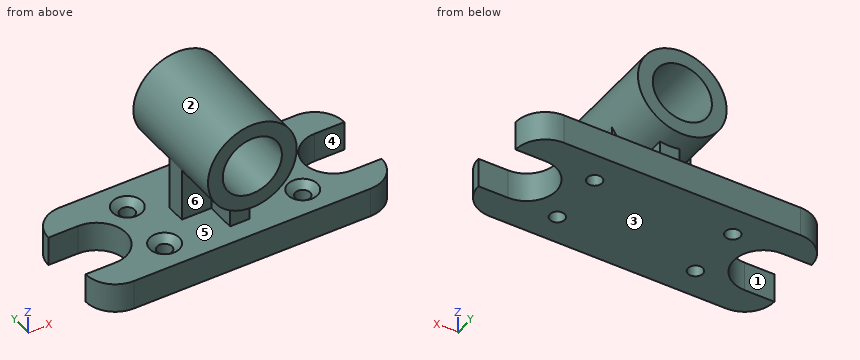
```python
from build123d import *

# Parameters (mm, degrees)
F0_R           = 38.1
F1_DEPTH       = 76.2
F2_DEPTH       = 266.7
F4_D           = 38.1
F4_CSINK_D     = 76.2
F4_CSINK_ANGLE = 100
F5_R           = 114.3
F5_R_2         = 76.2
F6_DEPTH       = 152.4
F7_DEPTH       = 152.4


with BuildPart() as f1:
    # F0 (on Top) → F1 (new body)
    with BuildSketch(Plane.XY):
        with BuildLine():
            ThreePointArc((-304.8, 76.2), (-228.6, 0), (-304.8, -76.2))
            Line((-304.8, -76.2), (-381, -76.2))
            ThreePointArc((-381, -76.2), (-358.681537, -130.081537), (-304.8, -152.4))
            Line((-304.8, -152.4), (304.8, -152.4))
            ThreePointArc((304.8, -152.4), (358.681537, -130.081537), (381, -76.2))
            Line((381, -76.2), (304.8, -76.2))
            ThreePointArc((304.8, -76.2), (228.6, 0), (304.8, 76.2))
            Line((304.8, 76.2), (381, 76.2))
            ThreePointArc((381, 76.2), (358.681537, 130.081537), (304.8, 152.4))
            Line((304.8, 152.4), (-304.8, 152.4))
            ThreePointArc((-304.8, 152.4), (-358.681537, 130.081537), (-381, 76.2))
            Line((-381, 76.2), (-304.8, 76.2))
        make_face()
        with Locations((-177.8, -76.2)):
            Circle(F0_R, mode=Mode.SUBTRACT)
        with Locations((177.8, -76.2)):
            Circle(F0_R, mode=Mode.SUBTRACT)
        with Locations((-177.8, 76.2)):
            Circle(F0_R, mode=Mode.SUBTRACT)
        Polygon((101.6, 25.4), (101.6, -25.4), (25.4, -25.4), (25.4, -101.6), (-25.4, -101.6), (-25.4, -25.4), (-101.6, -25.4), (-101.6, 25.4), (-25.4, 25.4), (-25.4, 101.6), (25.4, 101.6), (25.4, 25.4), align=None, mode=Mode.SUBTRACT)
        with Locations((177.8, 76.2)):
            Circle(F0_R, mode=Mode.SUBTRACT)
        with Locations((-177.8, 76.2)):
            Circle(F0_R)
        with Locations((-177.8, -76.2)):
            Circle(F0_R)
        with Locations((177.8, -76.2)):
            Circle(F0_R)
        with Locations((177.8, 76.2)):
            Circle(F0_R)
    extrude(amount=F1_DEPTH)

    # F0 (on Top) → F2 (join)
    with BuildSketch(Plane.XY):
        Polygon((25.4, -25.4), (101.6, -25.4), (101.6, 25.4), (25.4, 25.4), (25.4, 101.6), (-25.4, 101.6), (-25.4, 25.4), (-101.6, 25.4), (-101.6, -25.4), (-25.4, -25.4), (-25.4, -101.6), (25.4, -101.6), align=None)
    extrude(amount=F2_DEPTH)

    # F4 (through all)
    with Locations(Plane.XY.offset(76.2)):
        with Locations((-177.8, -76.2), (-177.8, 76.2), (177.8, 76.2), (177.8, -76.2)):
            CounterSinkHole(F4_D / 2, F4_CSINK_D / 2, counter_sink_angle=F4_CSINK_ANGLE)

    # F5 (on Front) → F6 (join, symmetric)
    with BuildSketch(Plane.XZ):
        with Locations((0, 266.7)):
            Circle(F5_R)
        with Locations((0, 266.7)):
            Circle(F5_R_2, mode=Mode.SUBTRACT)
    extrude(amount=F6_DEPTH, both=True)

    # F5 (on Front) → F7 (cut, symmetric)
    with BuildSketch(Plane.XZ):
        with Locations((0, 266.7)):
            Circle(F5_R_2)
    extrude(amount=F7_DEPTH, both=True, mode=Mode.SUBTRACT)


solid = f1.part
```
Verification items for the finished model (mm, model axes). Face numbers are marked on the shaded views. A direction names the side the tool comes from. Coordinates: 2 decimals unless noted, no trailing zeros. Write each loop counter-clockwise with the first axis right and the second up, starting at its lowest first coordinate (ties: lowest second). Pieces come first, ordered by that corner, then holes. Notation, with made-up numbers: M 46,83.5 L 60,83.5 A18 cw 60,98.5 Z; hole C 75.25,80.25 d9. An arc over 180 degrees is marked long. One line per item, written item: value.
Item 1: Section check A-A, the plane z = 266.7. Record the boundary of the cut face in (x, y).
Check sheet entries:
outline: M -114.3,-152.4 L -76.2,-152.4 L -76.2,152.4 L -114.3,152.4 Z; M 76.2,-152.4 L 114.3,-152.4 L 114.3,152.4 L 76.2,152.4 Z
Item 2: Section check D-D, the plane x = 18. Record the boundary of the cut face in (y, z), plus the area to 3 significant figures.
Check sheet entries:
outline: M -152.4,0 L 152.4,0 L 152.4,76.2 L 101.6,76.2 L 101.6,153.83 L 152.4,153.83 L 152.4,192.66 L -152.4,192.66 L -152.4,153.83 L -101.6,153.83 L -101.6,76.2 L -152.4,76.2 Z; M -152.4,340.74 L 152.4,340.74 L 152.4,379.57 L -152.4,379.57 Z
area: 62,700 mm^2
Item 3: Mould release check, pull along Z, two halves, no side actions. Record for the marked faces 1, 2 and 3: pulls with the +Z half, pulls with the -Z half, needs draft (parallel to the pull), parting line crosses it, or undercut.
Check sheet entries:
face 1: needs draft
face 2: undercut
face 3: pulls with the -Z half
Item 4: Access from +Z, -Z, +X, -X, +Y, -Y to the whole of each face (thin tool, end or side, straight path). Record for the marked faces 4, 5 and 6.
Check sheet entries:
face 4: +Z, -Z, +X
face 5: none
face 6: -X, -Y
Item 5: Gauge pin test, flat ends, axial feed: pin 1 Ø3 at (x, y) = (247.5, -99.5) entering from +Z; pin 2 Ø23 at (y, z) = (-69, 118.5) entering from +X; pin 3 Ø15 at (y, z) = (0, 125) entering from -X. Record the tip position at first contact, or that the pin passes through.
Check sheet entries:
pin 1: stops at z = 76.2
pin 2: stops at x = 25.4
pin 3: stops at x = -101.6
Item 6: Scan lines: line 1 along Y through (x, z) = (-177.8, 47); line 2 along X through (y, z) = (-96.5, 266); line 3 along X through (y, z) = (60, 42). Record each from-to range of solid material in increasing order.
Check sheet entries:
line 1: y = -152.4 to -95.25, -57.15 to 57.15, 95.25 to 152.4
line 2: x = -114.3 to -76.2, 76.2 to 114.3
line 3: x = -257.83 to -187.82, -167.78 to 167.78, 187.82 to 257.83
Item 7: Section check C-C, the plane y = 0. Record the boundary of the cut face in (x, z), plus the area to 3 significant figures.
Check sheet entries:
outline: M -228.6,0 L 228.6,0 L 228.6,76.2 L 101.6,76.2 L 101.6,214.34 A114.3 ccw long -101.6,214.34 L -101.6,76.2 L -228.6,76.2 Z; hole C 0,266.7 d152.4
area: 76,700 mm^2
Item 8: Section check B-B, the plane x = -177.8. Record the boundary of the cut face in (y, z).
Check sheet entries:
outline: M -152.4,0 L -95.25,0 L -95.25,60.22 L -114.3,76.2 L -152.4,76.2 Z; M -57.15,0 L 57.15,0 L 57.15,60.22 L 38.1,76.2 L -38.1,76.2 L -57.15,60.22 Z; M 95.25,0 L 152.4,0 L 152.4,76.2 L 114.3,76.2 L 95.25,60.22 Z
